Work out the finished part from the listing and answer in its coordinate system (mm). A direction names the side the tool comes from. Give positions to 0.01 mm unless a question says otherwise; leave off trailing zeros. Order: outer loops, then holes, each group sorted by start corner. A loop starts at its lowest first (then second) coordinate and runs counter-clockwise, first axis right, second up.
```python
from build123d import *

# Parameters (mm, degrees)
SKETCH1_W          = 100
SKETCH1_H          = 100
BASE_FLANGE1_DEPTH = 3
EDGE_FLANGE1_DEPTH = 100
EDGE_FLANGE2_DEPTH = 100
EDGE_FLANGE6_DEPTH = 100
EDGE_FLANGE7_DEPTH = 100


# Sheet-metal steps are written as plain solids
with BuildPart() as part:
    # Sketch1 → Base-Flange1 (new body)
    with BuildSketch(Plane.XY):
        Rectangle(SKETCH1_W, SKETCH1_H)
    extrude(amount=-BASE_FLANGE1_DEPTH)

    # Edge-Flange1 section (across the edge) → Edge-Flange1 (add)
    with BuildSketch(Plane(origin=(-53, 50, 0), x_dir=(1, 0, 0), z_dir=(0, -1, 0))):
        with BuildLine():
            Line((-3, 3), (-3, 37))
            Line((-3, 37), (0, 37))
            Line((0, 37), (0, 3))
            ThreePointArc((0, 3), (0.878679656, 0.878679656), (3, 0))
            Line((3, 0), (3, -3))
            ThreePointArc((3, -3), (-1.242640687, -1.242640687), (-3, 3))
        make_face()
    extrude(amount=EDGE_FLANGE1_DEPTH)

    # Edge-Flange2 section (across the edge) → Edge-Flange2 (add)
    with BuildSketch(Plane(origin=(53, -50, 0), x_dir=(-1, 0, 0), z_dir=(0, 1, 0))):
        with BuildLine():
            Line((-3, 3), (-3, 37))
            Line((-3, 37), (0, 37))
            Line((0, 37), (0, 3))
            ThreePointArc((0, 3), (0.878679656, 0.878679656), (3, 0))
            Line((3, 0), (3, -3))
            ThreePointArc((3, -3), (-1.242640687, -1.242640687), (-3, 3))
        make_face()
    extrude(amount=EDGE_FLANGE2_DEPTH)

    # Edge-Flange6 section (across the edge) → Edge-Flange6 (add)
    with BuildSketch(Plane(origin=(-53, 50, 40), x_dir=(0, 0, -1), z_dir=(0, -1, 0))):
        with BuildLine():
            Line((-3, 3), (-3, 22))
            Line((-3, 22), (0, 22))
            Line((0, 22), (0, 3))
            ThreePointArc((0, 3), (0.878679656, 0.878679656), (3, 0))
            Line((3, 0), (3, -3))
            ThreePointArc((3, -3), (-1.242640687, -1.242640687), (-3, 3))
        make_face()
    extrude(amount=EDGE_FLANGE6_DEPTH)

    # Edge-Flange7 section (across the edge) → Edge-Flange7 (add)
    with BuildSketch(Plane(origin=(53, -50, 40), x_dir=(0, 0, -1), z_dir=(0, 1, 0))):
        with BuildLine():
            Line((-3, 3), (-3, 17))
            Line((-3, 17), (0, 17))
            Line((0, 17), (0, 3))
            ThreePointArc((0, 3), (0.878679656, 0.878679656), (3, 0))
            Line((3, 0), (3, -3))
            ThreePointArc((3, -3), (-1.242640687, -1.242640687), (-3, 3))
        make_face()
    extrude(amount=EDGE_FLANGE7_DEPTH)


solid = part.part
```
1. The part is cut by section B-B (x = 39.5). Write down the section's boundary in (y, z), then the cut area to 3 significant figures.
Findings below:
outline: (-50, -3) - (50, -3) - (50, 0) - (-50, 0) - close; (-50, 40) - (50, 40) - (50, 43) - (-50, 43) - close
area: 600 mm2
2. The part is cut by section D-D (x = 13). Write down the section's boundary in (y, z).
Findings below:
outline: (-50, -3) - (50, -3) - (50, 0) - (-50, 0) - close
3. Straight lines are drawn through the part: probe 1 along Z at (x, y) = (-44, -44.5); probe 2 along X at (y, z) = (-42.5, 27.5); probe 3 along Z at (x, y) = (4, 33.5). For each, find the intervals that lie inside material, in ascending order.
Findings below:
probe 1: z = -3 to 0, 40 to 43
probe 2: x = -56 to -53, 53 to 56
probe 3: z = -3 to 0
4. The part is cut by section A-A (z = 20.5). Write down the section's boundary in (x, y).
Findings below:
outline: (-56, -50) - (-53, -50) - (-53, 50) - (-56, 50) - close; (53, -50) - (56, -50) - (56, 50) - (53, 50) - close
5. The part is cut by section C-C (y = -40.5). Write down the section's boundary in (x, z).
Findings below:
outline: (-56, 3) arc R6 ccw to (-50, -3) - (50, -3) arc R6 ccw to (56, 3) - (56, 37) arc R6 ccw to (50, 43) - (36, 43) - (36, 40) - (50, 40) arc R3 cw to (53, 37) - (53, 3) arc R3 cw to (50, 0) - (-50, 0) arc R3 cw to (-53, 3) - (-53, 37) arc R3 cw to (-50, 40) - (-31, 40) - (-31, 43) - (-50, 43) arc R6 ccw to (-56, 37) - close
6. The mould has two halves that part along X. Classify faces 4 (the face through (-31, 1, 42)), 5 (the face through (0, -50, -1)), 6 (the face through (54.196, -0.7, -1.289)): pulls with the +X half, pulls with the -X half, needs draft (parallel to the pull), parting line crosses it, or undercut.
Findings below:
face 4: undercut
face 5: needs draft
face 6: pulls with the +X half
7. Given P1, Ø8, axis at x = 1, y = 31.5, coming from the +Z side; P2, Ø1.5, axis at y = 0.5, z = 2, coming from the -X side; P3, Ø0.9, axis at y = -19.5, z = 41, coming from the +X side, each flat-ended and moving along its own axis, determine where each tip first touches the part or whether it passes through.
Findings below:
P1: stops at z = 0
P2: stops at x = -55.99
P3: stops at x = 54.84
8. Which of the six approach directions +Z, -Z, +X, -X, +Y, -Y give full straight-line access (tool end or side, diameter ignored) to faces 1 (the face through (-52.1, 0.7, 39.14)), 2 (the face through (54.289, -0.7, 41.196)), 3 (the face through (36, -1, 42))?
Findings below:
face 1: +Y, -Y
face 2: +Z, +X, +Y, -Y
face 3: +Z, +Y, -Y
